from build123d import *

# Parameters (mm, degrees)
SKETCH1_W                                      = 120
SKETCH1_H                                      = 90
BOSS_EXTRUDE1_DEPTH                            = 5
CSK_FOR_4_FLAT_HEAD_MACHINE_SCREW1_D           = 3.2639
CSK_FOR_4_FLAT_HEAD_MACHINE_SCREW1_CSINK_D     = 5.715
CSK_FOR_4_FLAT_HEAD_MACHINE_SCREW1_CSINK_ANGLE = 82
SKETCH5_R                                      = 2.5
SKETCH5_W                                      = 25
SKETCH5_H                                      = 72
CUT_EXTRUDE3_DEPTH                             = 76.166481892
SKETCH6_R                                      = 2
CUT_EXTRUDE4_DEPTH                             = 5


with BuildPart() as part:
    # Sketch1 → Boss-Extrude1 (new body)
    with BuildSketch(Plane(origin=(0, 0, 0), x_dir=(1, 0, 0), z_dir=(0, 1, 0))):
        Rectangle(SKETCH1_W, SKETCH1_H)
    extrude(amount=BOSS_EXTRUDE1_DEPTH)

    # CSK for #4 Flat Head Machine Screw1 (through all)
    with Locations(Plane(origin=(0, 0, 0), x_dir=(-1, 0, 0), z_dir=(0, -1, 0))):
        with Locations((-55, 40), (-55, -40), (55, -40), (55, 40)):
            CounterSinkHole(CSK_FOR_4_FLAT_HEAD_MACHINE_SCREW1_D / 2, CSK_FOR_4_FLAT_HEAD_MACHINE_SCREW1_CSINK_D / 2, counter_sink_angle=CSK_FOR_4_FLAT_HEAD_MACHINE_SCREW1_CSINK_ANGLE)

    # Sketch5 → Cut-Extrude3 (cut, through all)
    with BuildSketch(Plane(origin=(0, 5, 0), x_dir=(1, 0, 0), z_dir=(0, 1, 0))):
        with Locations(Location((0, -25, 0), (0, 0, 270))):
            Circle(SKETCH5_R)
        with Locations(Location((20, -25, 0), (0, 0, 270))):
            Circle(SKETCH5_R)
        with Locations(Location((40, -25, 0), (0, 0, 270))):
            Circle(SKETCH5_R)
        with Locations((-25.5, 0)):
            Rectangle(SKETCH5_W, SKETCH5_H)
    extrude(amount=-CUT_EXTRUDE3_DEPTH, mode=Mode.SUBTRACT)

    # Sketch6 → Cut-Extrude4 (cut)
    with BuildSketch(Plane(origin=(0, 5, 0), x_dir=(1, 0, 0), z_dir=(0, 1, 0))):
        with Locations(Location((0, 25, 0), (0, 0, 270))):
            Circle(SKETCH6_R)
    extrude(amount=-CUT_EXTRUDE4_DEPTH, mode=Mode.SUBTRACT)


solid = part.part
Work out the finished part from the listing and answer in its coordinate system (mm). A direction names the side the tool comes from. Give positions to 0.01 mm unless a question says otherwise; leave off trailing zeros. Write each loop counter-clockwise with the first axis right and the second up, starting at its lowest first coordinate (ties: lowest second). Pieces come first, ordered by that corner, then holes. Notation, with made-up numbers: (38.25, -27.5) - (95.25, -27.5) arc R20 cw to (95.25, -13.5) - close; hole circle Ø6 at (13, 53.5). An arc over 180 degrees is marked (long way). One line per item, written item: value. Start each with the question number.
1. Find section B-B (z = -25). Write down the section's boundary in (x, y), then the cut area to 3 significant figures.
2. Consider probe 1 along Z at (x, y) = (55, 3.7); probe 2 along X at (y, z) = (2.4, 40); probe 3 along X at (y, z) = (3.35, 25). Determine where each line is inside the solid, lowest interval first.
3. Find section D-D (z = 25). Write down the section's boundary in (x, y), then the cut area to 3 significant figures.
4. For faces 4 (the flat face through (-38, 3, 1)), 5 (the flat face through (-1, 5, -1)), determine the directions among +Z, -Z, +X, -X, +Y, -Y from which every point of the face is accessible in a straight line to the end or side of a thin tool.
5. Find section A-A (x = 55). Write down the section's boundary in (y, z).
6. Find section C-C (x = 40). Write down the section's boundary in (y, z), then the cut area to 3 significant figures.
7. Given pin 1 (6 mm diameter, centred on x = 29.5, z = 10, fed in from -Y); pin 2 (5 mm diameter, centred on x = -55, z = -40, fed in from -Y); pin 3 (4 mm diameter, centred on x = -55, z = 40, fed in from -Y), each flat-ended and moving along its own axis, determine where each tip first touches the part or whether it passes through.
8. For a pull along X with two mould halves and no side action, classify faces 1 (the flat face through (-1, 2, 45)), 2 (the flat face through (-26, 3, -36)), 3 (the flat face through (-60, 2, 1)) as +X half, -X half, draft (parallel to the pull), parting line (faces both ways), or undercut.
Geometry results:
1. outline: (-60, 0) - (-38, 0) - (-38, 5) - (-60, 5) - close; (-13, 0) - (-2, 0) - (-2, 5) - (-13, 5) - close; (2, 0) - (60, 0) - (60, 5) - (2, 5) - close
1. area: 455 mm2
2. probe 1: -45 to -41.63, -38.37 to 38.37, 41.63 to 45
2. probe 2: -60 to -56.63, -53.37 to 53.37, 56.63 to 60
2. probe 3: -60 to -38, -13 to -2.5, 2.5 to 17.5, 22.5 to 37.5, 42.5 to 60
3. outline: (-60, 0) - (-38, 0) - (-38, 5) - (-60, 5) - close; (-13, 0) - (-2.5, 0) - (-2.5, 5) - (-13, 5) - close; (2.5, 0) - (17.5, 0) - (17.5, 5) - (2.5, 5) - close; (22.5, 0) - (37.5, 0) - (37.5, 5) - (22.5, 5) - close; (42.5, 0) - (60, 0) - (60, 5) - (42.5, 5) - close
3. area: 400 mm2
4. face 4: +Y, -Y
4. face 5: +Z, -Z, +X, -X, +Y
5. outline: (0, -45) - (5, -45) - (5, -41.63) - (1.41, -41.63) - (0, -42.86) - close; (0, -37.14) - (1.41, -38.37) - (5, -38.37) - (5, 38.37) - (1.41, 38.37) - (0, 37.14) - close; (0, 42.86) - (1.41, 41.63) - (5, 41.63) - (5, 45) - (0, 45) - close
6. outline: (0, -45) - (5, -45) - (5, 22.5) - (0, 22.5) - close; (0, 27.5) - (5, 27.5) - (5, 45) - (0, 45) - close
6. area: 425 mm2
7. pin 1: y = 0
7. pin 2: y = 0.41
7. pin 3: y = 0.99
8. face 1: draft
8. face 2: undercut
8. face 3: -X half
